Read the model definition and answer for the solid it produces. Units are mm, in the model's axes. Coordinates: 2 decimals unless noted, no trailing zeros. Loops run counter-clockwise (first coordinate to the right, second up) from the corner with the lowest first, then second, coordinate; pieces in that order, holes last. Notation, with made-up numbers: M -21.75,24 L -5.75,24 A27 ccw -5.75,42 Z; hole C 18,17 d4. An arc over 180 degrees is marked long. One line per item, written item: value. Start each with the question number.
```python
from build123d import *

# Parameters (mm, degrees)
SKETCH1_R           = 22
BOSS_EXTRUDE1_DEPTH = 3.175
SKETCH4_R           = 1.745
CUT_EXTRUDE2_DEPTH  = 32.274280567
SKETCH2_R           = 6.45
CUT_EXTRUDE4_DEPTH  = 32.274280567
CIRPATTERN1_COUNT   = 8
SKETCH5_R           = 3.175
CUT_EXTRUDE5_DEPTH  = 32.274280567
CIRPATTERN2_COUNT   = 4


with BuildPart() as part:
    # Sketch1 → Boss-Extrude1 (new body)
    with BuildSketch(Plane(origin=(0, 0, 0), x_dir=(1, 0, 0), z_dir=(0, 1, 0))):
        with Locations(Location((0, 0, 0), (0, 0, 270))):
            Circle(SKETCH1_R)
    extrude(amount=-BOSS_EXTRUDE1_DEPTH)

    # Sketch4 → Cut-Extrude2 (cut, symmetric)
    with BuildSketch(Plane(origin=(0, 0, 0), x_dir=(1, 0, 0), z_dir=(0, 1, 0))):
        with Locations(Location((0, -9.779, 0), (0, 0, 270))):
            Circle(SKETCH4_R)
    cut_extrude2 = extrude(amount=CUT_EXTRUDE2_DEPTH, both=True, mode=Mode.SUBTRACT)

    # Sketch2 → Cut-Extrude4 (cut, through all)
    with BuildSketch(Plane(origin=(0, 0, 0), x_dir=(1, 0, 0), z_dir=(0, 1, 0))):
        with Locations(Location((0, 0, 0), (0, 0, 270))):
            Circle(SKETCH2_R)
    extrude(amount=-CUT_EXTRUDE4_DEPTH, mode=Mode.SUBTRACT)

    # CirPattern1: Cut-Extrude2 ×8 about axis
    cirpattern1_axis = Axis((0, 0, 0), (0, 1, 0))
    for i in range(1, CIRPATTERN1_COUNT):
        add(cut_extrude2.rotate(cirpattern1_axis, i * 360 / CIRPATTERN1_COUNT), mode=Mode.SUBTRACT)

    # Sketch5 → Cut-Extrude5 (cut, through all)
    with BuildSketch(Plane(origin=(0, 0, 0), x_dir=(1, 0, 0), z_dir=(0, 1, 0))):
        with Locations(Location((6.50561835, 15.705952053, 0), (0, 0, 270))):
            Circle(SKETCH5_R)
    cut_extrude5 = extrude(amount=-CUT_EXTRUDE5_DEPTH, mode=Mode.SUBTRACT)

    # CirPattern2: Cut-Extrude5 ×4 about axis
    cirpattern2_axis = Axis((0, 0, 0), (0, 1, 0))
    for i in range(1, CIRPATTERN2_COUNT):
        add(cut_extrude5.rotate(cirpattern2_axis, i * 360 / CIRPATTERN2_COUNT), mode=Mode.SUBTRACT)


solid = part.part
```
1) Flat-ended cylindrical pins translate along their axes: pin 1 (3 mm diameter, centred on x = 6.91, z = -6.91, fed in from -Y); pin 2 (1.5 mm diameter, centred on y = -1, z = 5.5, fed in from -X); pin 3 (1.5 mm diameter, centred on y = -2, z = 12.5, fed in from -X). Find the tip coordinate at first contact, or state that the pin passes through.
2) Section A-A (z = 0) is taken. Determine the outline of the cut face in (x, y) (3 decimals), then the cut area to 3 significant figures.
3) Section C-C (x = -15.5) is taken. Determine the outline of the cut face in (y, z) (1 decimal), then the cut area to 3 significant figures.
4) For a pull along Z with two mould halves and no side action, classify faces 1 (the face through (-21.477, -1.565, -4.769)), 2 (the face through (-11.39, -1.57, -0.67)), 3 (the face through (-5, 0, 5)) as released by +Z, released by -Z, zero draft, split by the parting line, or undercut.
5) Consider line 1 along Z through (x, y) = (-8, -1); line 2 along X through (y, z) = (-2.25, 5); line 3 along Z through (x, y) = (1.5, -1.95). Determine where each line is inside the solid, lowest interval first.
6) Section B-B (x = 0) is taken. Determine the outline of the cut face in (y, z) (3 decimals).
7) Section D-D (z = -14) is taken. Determine the outline of the cut face in (x, y) (3 decimals).
Results found:
1. pin 1: passes through
1. pin 2: stops at x = -21.48
1. pin 3: stops at x = -18.6
2. outline: M -22,-3.175 L -11.524,-3.175 L -11.524,0 L -22,0 Z; M -8.034,-3.175 L -6.45,-3.175 L -6.45,0 L -8.034,0 Z; M 6.45,-3.175 L 8.034,-3.175 L 8.034,0 L 6.45,0 Z; M 11.524,-3.175 L 22,-3.175 L 22,0 L 11.524,0 Z
2. area: 76.6 mm²
3. outline: M -3.2,-15.6 L 0,-15.6 L 0,-9.7 L -3.2,-9.7 Z; M -3.2,-3.3 L 0,-3.3 L 0,15.6 L -3.2,15.6 Z
3. area: 79.0 mm²
4. face 1: split by the parting line
4. face 2: undercut
4. face 3: zero draft
5. line 1: z = -20.49 to -8.28, -5.55 to 5.55, 8.28 to 12.9, 18.51 to 20.49
5. line 2: x = -21.42 to -4.07, 4.07 to 12.91, 18.5 to 21.42
5. line 3: z = -21.95 to -10.67, -8.89 to -6.27, 6.27 to 8.89, 10.67 to 21.95
6. outline: M -3.175,-22 L 0,-22 L 0,-11.524 L -3.175,-11.524 Z; M -3.175,-8.034 L 0,-8.034 L 0,-6.45 L -3.175,-6.45 Z; M -3.175,6.45 L 0,6.45 L 0,8.034 L -3.175,8.034 Z; M -3.175,11.524 L 0,11.524 L 0,22 L -3.175,22 Z
7. outline: M -16.971,-3.175 L 3.828,-3.175 L 3.828,0 L -16.971,0 Z; M 9.183,-3.175 L 16.971,-3.175 L 16.971,0 L 9.183,0 Z
